Geometry: final body of the model. Coordinates: model frame, mm. A direction names the side the tool comes from. Coordinates: 2 decimals unless noted, no trailing zeros. Loops run counter-clockwise (first coordinate to the right, second up) from the corner with the lowest first, then second, coordinate; pieces in that order, holes last. Notation, with made-up numbers: (-21, 76) - (35, 76) arc R18 cw to (35, 83) - close; hole circle Ø6 at (9.25, -6.75). An arc over 180 degrees is marked (long way). Answer in a Markdown table with one row per item.
from build123d import *

# Parameters (mm, degrees)
BOSS_EXTRUDE1_DEPTH = 19.05


with BuildPart() as part:
    # Sketch1 → Boss-Extrude1 (new body)
    with BuildSketch(Plane(origin=(0, 0, 0), x_dir=(1, 0, 0), z_dir=(0, 1, 0))):
        with BuildLine():
            Line((-108.53449825, -3.903212814), (-108.53449825, 1464.036274944))
            ThreePointArc((-108.53449825, 1464.036274944), (-109.501228187, 1468.896354535), (-112.254242128, 1473.016531065))
            Line((-112.254242128, 1473.016531065), (-511.214754371, 1871.977043307))
            ThreePointArc((-511.214754371, 1871.977043307), (-515.334930901, 1874.730057249), (-520.195010492, 1875.696787186))
            Line((-520.195010492, 1875.696787186), (-756.23449825, 1875.696787186))
            ThreePointArc((-756.23449825, 1875.696787186), (-765.214754371, 1871.977043307), (-768.93449825, 1862.996787186))
            Line((-768.93449825, 1862.996787186), (-768.93449825, 1680.674485719))
            ThreePointArc((-768.93449825, 1680.674485719), (-766.912332227, 1673.798886723), (-761.489795642, 1669.112831455))
            Line((-761.489795642, 1669.112831455), (-638.63184093, 1613.268306586))
            ThreePointArc((-638.63184093, 1613.268306586), (-632.516703345, 1607.363790151), (-631.495541921, 1598.924865375))
            Line((-631.495541921, 1598.924865375), (-768.93449825, 986.696787186))
            Line((-768.93449825, 986.696787186), (-768.93449825, 834.296787186))
            Line((-768.93449825, 834.296787186), (-972.13449825, 834.296787186))
            Line((-972.13449825, 834.296787186), (-972.13449825, 737.957299428))
            ThreePointArc((-972.13449825, 737.957299428), (-971.167768312, 733.097219837), (-968.414754371, 728.977043307))
            Line((-968.414754371, 728.977043307), (-874.254242128, 634.816531065))
            ThreePointArc((-874.254242128, 634.816531065), (-871.501228187, 630.696354535), (-870.53449825, 625.836274944))
            Line((-870.53449825, 625.836274944), (-870.53449825, -3.903212814))
            Line((-870.53449825, -3.903212814), (-108.53449825, -3.903212814))
        make_face()
    extrude(amount=BOSS_EXTRUDE1_DEPTH)


solid = part.part
(1) Cut plane C-C on z = -140. Output: boundary loops of the cut face in (x, y).
Verdict:
| item | result |
|---|---|
| outline | (-870.53, 0) - (-108.53, 0) - (-108.53, 19.05) - (-870.53, 19.05) - close |
(2) Cut plane D-D on x = -245. Output: boundary loops of the cut face in (y, z).
Verdict:
| item | result |
|---|---|
| outline | (0, -1605.76) - (19.05, -1605.76) - (19.05, 3.9) - (0, 3.9) - close |
(3) Ray query, probe 1 along Z at (x, y) = (-804, 1.75); probe 2 along X at (y, z) = (9.75, -557); probe 3 along X at (y, z) = (2, -962). Return the intervals inside material, ascending.
Verdict:
| item | result |
|---|---|
| probe 1 | z = -834.3 to 3.9 |
| probe 2 | x = -870.53 to -108.53 |
| probe 3 | x = -768.93 to -108.53 |
(4) Pull-direction query (Z, two-part tool) for faces 3 (the face through (-699.253, 9.392, -1297.096)), 4 (the face through (-450, 19.05, -740)), 5 (the face through (-921.994, 9.392, -682.556)); classes: pulls with the +Z half, pulls with the -Z half, needs draft (parallel to the pull), parting line crosses it, or undercut.
Verdict:
| item | result |
|---|---|
| face 3 | undercut |
| face 4 | needs draft |
| face 5 | pulls with the +Z half |
(5) Cut plane A-A on x = -664. Output: boundary loops of the cut face in (y, z).
Verdict:
| item | result |
|---|---|
| outline | (0, -1875.7) - (19.05, -1875.7) - (19.05, -1624.8) - (0, -1624.8) - close; (0, -1454.13) - (19.05, -1454.13) - (19.05, 3.9) - (0, 3.9) - close |
(6) Cut plane B-B on y = 14.75. Output: boundary loops of the cut face in (x, z), then the cut area to 3 significant figures.
Verdict:
| item | result |
|---|---|
| outline | (-972.13, -834.3) - (-768.93, -834.3) - (-768.93, -986.7) - (-631.5, -1598.92) arc R12.7 cw to (-638.63, -1613.27) - (-761.49, -1669.11) arc R12.7 ccw to (-768.93, -1680.67) - (-768.93, -1863) arc R12.7 ccw to (-756.23, -1875.7) - (-520.2, -1875.7) arc R12.7 ccw to (-511.21, -1871.98) - (-112.25, -1473.02) arc R12.7 ccw to (-108.53, -1464.04) - (-108.53, 3.9) - (-870.53, 3.9) - (-870.53, -625.84) arc R12.7 cw to (-874.25, -634.82) - (-968.41, -728.98) arc R12.7 ccw to (-972.13, -737.96) - close |
| area | 1,210,000 mm² |
(7) First-contact query: pin 1 Ø2 at (x, z) = (-580.5, -995.5) entering from -Y; pin 2 Ø4 at (x, y) = (-346, 15.5) entering from -Z; pin 3 Ø1 at (y, z) = (4.5, -1340.5) entering from -X; pin 4 Ø10 at (y, z) = (9, -1641.5) entering from +X. Flat tips, straight axial feed; report the tip coordinate or a pass-through.
Verdict:
| item | result |
|---|---|
| pin 1 | stops at y = 0 |
| pin 2 | stops at z = -1708.76 |
| pin 3 | stops at x = -689.62 |
| pin 4 | stops at x = -275.74 |
(8) Access query for faces 1 (the face through (-700.92, 9.39, -1641.58)), 2 (the face through (-308.94, 9.39, -1669.7)). Directions: +Z, -Z, +X, -X, +Y, -Y. A direction counts if a zero-diameter tool reaches every point of the face in a straight line with its end or side. Return the directions, or none.
Verdict:
| item | result |
|---|---|
| face 1 | -X, +Y, -Y |
| face 2 | -Z, +X, +Y, -Y |
